Geometry check sheet. Reference: the model listing, model coordinates, mm. Face numbers are marked on the shaded views. A direction names the side the tool comes from. Round coordinates to 2 decimals unless told otherwise and drop trailing zeros. Write each loop counter-clockwise with the first axis right and the second up, starting at its lowest first coordinate (ties: lowest second). Pieces come first, ordered by that corner, then holes. Notation, with made-up numbers: M -25,75 L 17,75 A21 ccw 17,89 Z; hole C 42,33.5 d4. An arc over 180 degrees is marked long. Use a Markdown table: item, result.
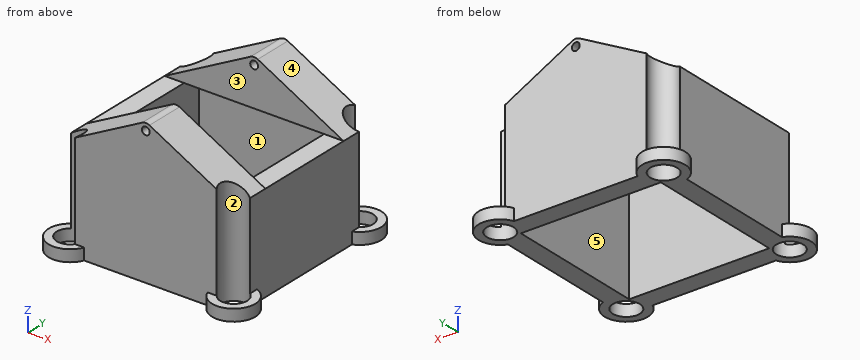
```python
from build123d import *

# Parameters (mm, degrees)
F0_R      = 1.65
F1_DEPTH  = 25
F4_DEPTH  = 23
F7_DEPTH  = 13
F5_R      = 3.466922
F8_DEPTH  = 36
F6_R      = 5.544206
F6_R_2    = 3.466922
F9_DEPTH  = 3
F2_W      = 36
F2_H      = 36
F10_DEPTH = 25
F11_R     = 2


with BuildPart() as f1:
    # F0 (on Top) → F1 (new body)
    with BuildSketch(Plane.XY):
        Polygon((23, 23), (0, 23), (-23, 23), (-23, 0), (-23, -23), (0, -23), (23, -23), (23, 0), align=None)
        with Locations((-20.221745, -20.221745)):
            Circle(F0_R, mode=Mode.SUBTRACT)
        with Locations((20.221745, -20.221745)):
            Circle(F0_R, mode=Mode.SUBTRACT)
        with Locations((-20.221745, 20.221745)):
            Circle(F0_R, mode=Mode.SUBTRACT)
        with Locations((20.221745, 20.221745)):
            Circle(F0_R, mode=Mode.SUBTRACT)
    extrude(amount=F1_DEPTH)

    # F3 (on Front) → F4 (join, symmetric)
    with BuildSketch(Plane.XZ):
        Polygon((-23, 25), (0, 25), (23, 25), (0, 37.124356), align=None)
        with BuildLine():
            ThreePointArc((0, 36.037711), (1, 35.037711), (0, 34.037711))
            ThreePointArc((0, 34.037711), (-1, 35.037711), (0, 36.037711))
        make_face(mode=Mode.SUBTRACT)
    extrude(amount=F4_DEPTH, both=True)

    # F3 (on Front) → F7 (cut, symmetric)
    with BuildSketch(Plane.XZ):
        Polygon((-23, 25), (0, 25), (23, 25), (0, 37.124356), align=None)
        with BuildLine():
            ThreePointArc((0, 36.037711), (1, 35.037711), (0, 34.037711))
            ThreePointArc((0, 34.037711), (-1, 35.037711), (0, 36.037711))
        make_face(mode=Mode.SUBTRACT)
    extrude(amount=F7_DEPTH, both=True, mode=Mode.SUBTRACT)

    # F5 (on Top) → F8 (cut)
    with BuildSketch(Plane.XY):
        with Locations((-21.004396, 20.949436)):
            Circle(F5_R)
        with Locations((21.004396, 20.949436)):
            Circle(F5_R)
        with Locations((21.004396, -20.949436)):
            Circle(F5_R)
        with Locations((-21.004396, -20.949436)):
            Circle(F5_R)
    extrude(amount=F8_DEPTH, mode=Mode.SUBTRACT)

    # F6 (on Top) → F9 (join)
    with BuildSketch(Plane.XY):
        with Locations((-21.004396, 20.949436)):
            Circle(F6_R)
        with Locations((-21.004396, 20.949436)):
            Circle(F6_R_2, mode=Mode.SUBTRACT)
        with Locations((21.004396, 20.949436)):
            Circle(F6_R)
        with Locations((21.004396, 20.949436)):
            Circle(F6_R_2, mode=Mode.SUBTRACT)
        with Locations((21.004396, -20.949436)):
            Circle(F6_R)
        with Locations((21.004396, -20.949436)):
            Circle(F6_R_2, mode=Mode.SUBTRACT)
        with Locations((-21.004396, -20.949436)):
            Circle(F6_R)
        with Locations((-21.004396, -20.949436)):
            Circle(F6_R_2, mode=Mode.SUBTRACT)
    extrude(amount=F9_DEPTH)

    # F2 (on face) → F10 (cut)
    with BuildSketch(Plane(origin=(0, 0, 0), x_dir=(1, 0, 0), z_dir=(0, 0, -1))):
        Rectangle(F2_W, F2_H)
    extrude(amount=-F10_DEPTH, mode=Mode.SUBTRACT)

    # F11
    f11_edges = [f1.edges().sort_by_distance(p)[0] for p in [
        (0, 18, 37.124356),
        (0, -18, 37.124356),
    ]]
    fillet(f11_edges, radius=F11_R)


solid = f1.part
```
Item 1: Cross-section at C-C, the plane y = -7. Record the cut outline in (x, z), and give its area (3 significant figures).
Outcome:
| item | result |
|---|---|
| outline | M -23,0 L -18,0 L -18,25 L -23,25 Z; M 18,0 L 23,0 L 23,25 L 18,25 Z |
| area | 250 mm2 |
Item 2: Mould release check, pull along X, two halves, no side actions. Record for the marked faces 3, 4 and 5: +X half, -X half, draft (parallel to the pull), parting line (faces both ways), or undercut.
Outcome:
| item | result |
|---|---|
| face 3 | draft |
| face 4 | +X half |
| face 5 | undercut |
Item 3: Cross-section at B-B, the plane z = 19. Record the cut outline in (x, y), and give its area (3 significant figures).
Outcome:
| item | result |
|---|---|
| outline | M -23,-18.11 A3.47 cw -18.21,-23 L 18.21,-23 A3.47 cw 23,-18.11 L 23,18.11 A3.47 cw 18.21,23 L -18.21,23 A3.47 cw -23,18.11 Z; hole M -18,-18 L 18,-18 L 18,18 L -18,18 Z |
| area | 713 mm2 |
Item 4: Cross-section at D-D, the plane x = -22. Record the cut outline in (y, z), and give its area (3 significant figures).
Outcome:
| item | result |
|---|---|
| outline | M -26.4,0 L -24.27,0 L -24.27,3 L -26.4,3 Z; M -17.63,0 L 17.63,0 L 17.63,25.53 L 13,25.53 L 13,25 L -13,25 L -13,25.53 L -17.63,25.53 Z; M 24.27,0 L 26.4,0 L 26.4,3 L 24.27,3 Z |
| area | 899 mm2 |
Item 5: Cross-section at A-A, the plane x = 0. Record the cut outline in (y, z), and give its area (3 significant figures).
Outcome:
| item | result |
|---|---|
| outline | M -23,0 L -18,0 L -18,25 L -13,25 L -13,34.04 L -23,34.04 Z; M -23,36.04 L -13,36.04 L -13,36.86 L -23,36.86 Z; M 13,25 L 18,25 L 18,0 L 23,0 L 23,34.04 L 13,34.04 Z; M 13,36.04 L 23,36.04 L 23,36.86 L 13,36.86 Z |
| area | 447 mm2 |
Item 6: Material ranges on line 1 along X through (y, z) = (4, 14); line 2 along Y through (x, z) = (-19.5, 26.5), recorded low to high. Write a range as from..to.
Outcome:
| item | result |
|---|---|
| line 1 | x = -23..-18, 18..23 |
| line 2 | y = -17.83..-13, 13..17.83 |
Item 7: Access from +Z, -Z, +X, -X, +Y, -Y to the whole of each face (thin tool, end or side, straight path). Record for the marked faces 1 and 2.
Outcome:
| item | result |
|---|---|
| face 1 | -Z |
| face 2 | +Z, -Z |
Item 8: Go/stop test with flat-tipped pins: pin 1 (7.5 mm diameter, centred on x = -7.5, z = 7.5, fed in from +Y); pin 2 (8.5 mm diameter, centred on x = 19, y = -19.5, fed in from +Z); pin 3 (7.5 mm diameter, centred on y = -4, z = 12.5, fed in from +X). Record where each tip stops, or that it passes through.
Outcome:
| item | result |
|---|---|
| pin 1 | stops at y = 23 |
| pin 2 | stops at z = 29.35 |
| pin 3 | stops at x = 23 |
